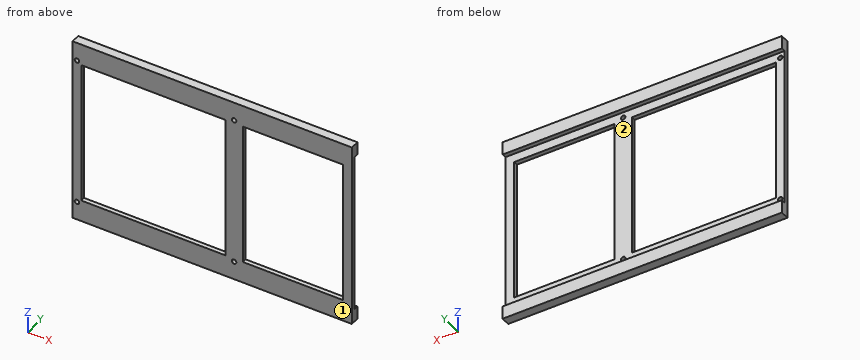
from build123d import *

# Parameters (mm, degrees)
SKETCH1_W                 = 203.2
SKETCH1_H                 = 136.398
BOSS_EXTRUDE1_DEPTH       = 6.35
SKETCH3_W                 = 117.348
SKETCH3_H                 = 3.175
CUT_EXTRUDE1_DEPTH        = 204.2
SKETCH4_W                 = 104.775
SKETCH4_H                 = 104.648
SKETCH4_W_2               = 73.025
CUT_EXTRUDE3_DEPTH        = 4.175
M4X0_7_TAPPED_HOLE1_D     = 3.3
M4X0_7_TAPPED_HOLE1_DEPTH = 9.906


with BuildPart() as part:
    # Sketch1 → Boss-Extrude1 (new body)
    with BuildSketch(Plane(origin=(0, 0, 0), x_dir=(1, 0, 0), z_dir=(0, 1, 0))):
        Rectangle(SKETCH1_W, SKETCH1_H)
    extrude(amount=BOSS_EXTRUDE1_DEPTH)

    # Sketch3 → Cut-Extrude1 (cut, through all)
    with BuildSketch(Plane(origin=(101.6, 0, 0), x_dir=(0, 0, -1), z_dir=(1, 0, 0))):
        with Locations((0, 4.7625)):
            Rectangle(SKETCH3_W, SKETCH3_H)
    extrude(amount=-CUT_EXTRUDE1_DEPTH, mode=Mode.SUBTRACT)

    # Sketch4 → Cut-Extrude3 (cut, through all)
    with BuildSketch(Plane(origin=(0, 3.175, 0), x_dir=(1, 0, 0), z_dir=(0, 1, 0))):
        with Locations((-42.8625, 0)):
            Rectangle(SKETCH4_W, SKETCH4_H)
        with Locations((58.7375, 0)):
            Rectangle(SKETCH4_W_2, SKETCH4_H)
    extrude(amount=-CUT_EXTRUDE3_DEPTH, mode=Mode.SUBTRACT)

    # M4x0.7 Tapped Hole1
    with Locations(Plane(origin=(0, 3.175, 0), x_dir=(1, 0, 0), z_dir=(0, 1, 0))):
        with Locations((-98.425, -54.61), (-98.425, 54.61), (15.875, 54.61), (15.875, -54.61)):
            Hole(M4X0_7_TAPPED_HOLE1_D / 2, depth=M4X0_7_TAPPED_HOLE1_DEPTH)


solid = part.part
The model under review builds one solid part; all positions refer to its coordinate system, in mm. Face numbers are marked on the shaded views. Give positions to 0.01 mm unless a question says otherwise; leave off trailing zeros. Order: outer loops, then holes, each group sorted by start corner. A loop starts at its lowest first (then second) coordinate and runs counter-clockwise, first axis right, second up. Notation, with made-up numbers: M 20.25,17 L 62.25,17 A13 ccw 62.25,40 Z; hole C 85,0 d8. An arc over 180 degrees is marked long. Use one line per item in the form item = value. Start each with the question number.
Item 1: Insertion check: pin 1 Ø3 at (x, z) = (15.875, -54.61) entering from +Y. The pin has a flat end and moves straight along its axis. Give the tip position at first contact, or say it passes through.
Item 2: The part is to be moulded in two halves that separate along Z. For the marked faces 1 and 2, say which applies: pulls with the +Z half, pulls with the -Z half, needs draft (parallel to the pull), parting line crosses it, or undercut.
Item 3: We need section B-B on y = 4.5. Give the boundary of the cut face in (x, z).
Item 4: We need section A-A on z = -11. Give the boundary of the cut face in (x, y) (3 decimals).
Item 5: To check wall thickness, follow line 1 along X through (y, z) = (2.5, -54.61) (3 decimals); line 2 along X through (y, z) = (1.5, -21) (3 decimals); line 3 along Z through (x, y) = (-44, 1). State the ranges of each line that lie inside material, in increasing order. Write a range as from..to.
Item 6: We need section C-C on x = 6. Give the boundary of the cut face in (y, z) (3 decimals), plus the area to 3 significant figures.
Completed:
q1.pin_1 = through
q2.face_1 = needs draft
q2.face_2 = undercut
q3.outline = M -101.6,-68.2 L 101.6,-68.2 L 101.6,-58.67 L -101.6,-58.67 Z; M -101.6,58.67 L 101.6,58.67 L 101.6,68.2 L -101.6,68.2 Z
q4.outline = M -101.6,0 L -95.25,0 L -95.25,3.175 L -101.6,3.175 Z; M 9.525,0 L 22.225,0 L 22.225,3.175 L 9.525,3.175 Z; M 95.25,0 L 101.6,0 L 101.6,3.175 L 95.25,3.175 Z
q5.line_1 = -101.6..-100.075, -96.775..14.225, 17.525..101.6
q5.line_2 = -101.6..-95.25, 9.525..22.225, 95.25..101.6
q5.line_3 = -68.2..-52.32, 52.32..68.2
q6.outline = M 0,-68.199 L 6.35,-68.199 L 6.35,-58.674 L 3.175,-58.674 L 3.175,-52.324 L 0,-52.324 Z; M 0,52.324 L 3.175,52.324 L 3.175,58.674 L 6.35,58.674 L 6.35,68.199 L 0,68.199 Z
q6.area = 161 mm²
